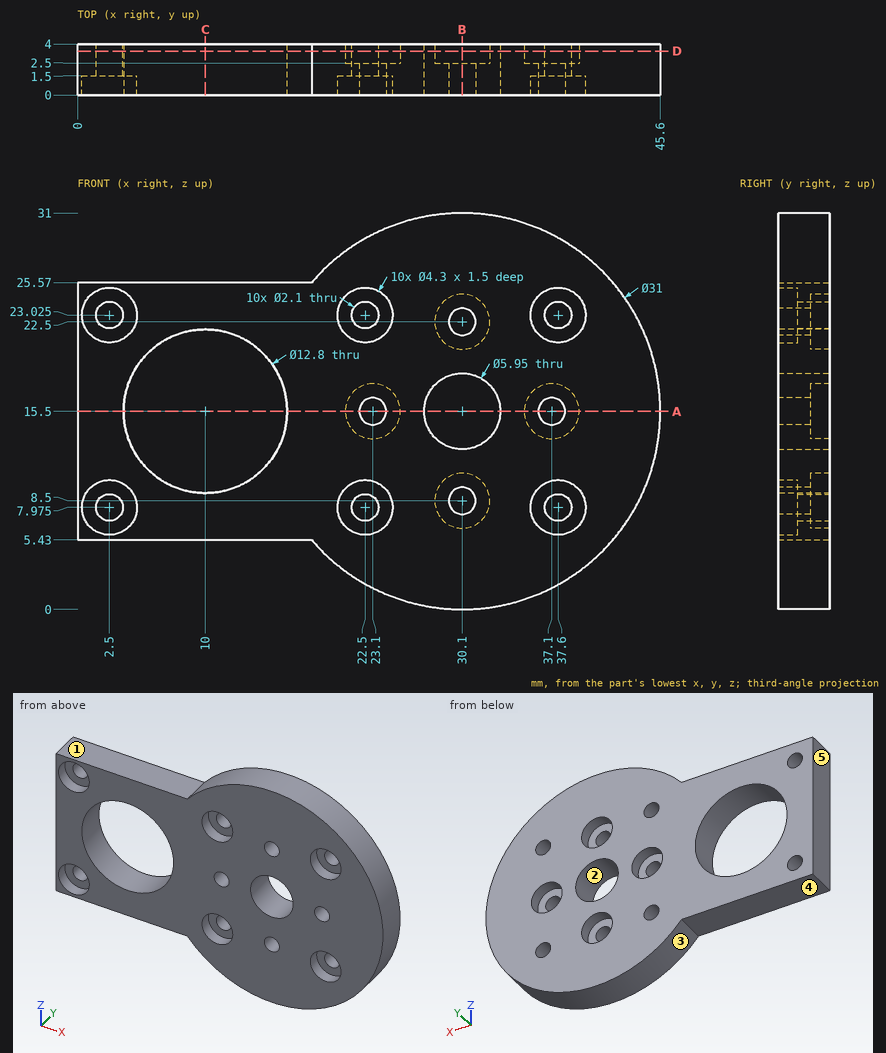
Geometry: see drawing. Coordinates: mm, zero at the bounding-box minimum. A direction names the side the tool comes from. Give positions to 0.01 mm unless a question says otherwise; leave off trailing zeros. Write each loop counter-clockwise with the first axis right and the second up, starting at its lowest first coordinate (ties: lowest second). Pieces come first, ordered by that corner, then holes. Notation, with made-up numbers: M 10,27 L 56,27 A34 cw 56,64 Z; hole C 81.5,51.25 d3. An arc over 180 degrees is marked long. Answer as a JSON object with one key per item and string values.
Q1. Contact query for flat-ended pins moving along their axis: P1, Ø1.3, axis at x = 37.5, z = 22, coming from the -Y side; P2, Ø1.3, axis at x = 2.5, z = 7.975, coming from the +Y side; P3, Ø2, axis at x = 29.5, z = 8, coming from the +Y side. Output: stop coordinate, or through.
Geometry check:
{"P1": "stops at y = 1.5", "P2": "passes through", "P3": "stops at y = 2.5"}
Q2. Cut plane B-B, the plane x = 30.1. Return the cut outline in (y, z) (3 decimals), then the cut area to 3 significant figures.
Geometry check:
{"outline": "M 0,0 L 4,0 L 4,6.35 L 2.5,6.35 L 2.5,7.45 L 0,7.45 Z; M 0,9.55 L 2.5,9.55 L 2.5,10.65 L 4,10.65 L 4,12.525 L 0,12.525 Z; M 0,18.475 L 4,18.475 L 4,20.35 L 2.5,20.35 L 2.5,21.45 L 0,21.45 Z; M 0,23.55 L 2.5,23.55 L 2.5,24.65 L 4,24.65 L 4,31 L 0,31 Z", "area": "76.8 mm^2"}
Q3. Ray query, line 1 along X through (y, z) = (0.8, 15.5) (3 decimals); line 2 along Z through (x, y) = (10, 3.25); line 3 along X through (y, z) = (0.2, 17.5). Return the intervals inside material, ascending.
Geometry check:
{"line 1": "x = 0 to 3.6, 16.4 to 22.05, 24.15 to 27.125, 33.075 to 36.05, 38.15 to 45.6", "line 2": "z = 5.43 to 9.1, 21.9 to 25.57", "line 3": "x = 0 to 3.92, 16.08 to 27.9, 32.3 to 45.47"}
Q4. Access query for the marked faces 4 and 5. Directions: +Z, -Z, +X, -X, +Y, -Y. A direction counts if a zero-diameter tool reaches every point of the face in a straight line with its end or side. Return the directions, or none.
Geometry check:
{"face 4": "-Z, -X, +Y, -Y", "face 5": "+Z, -Z, -X, +Y, -Y"}
Q5. Cut plane A-A, the plane z = 15.5. Return the cut outline in (x, y) (3 decimals).
Geometry check:
{"outline": "M 0,0 L 3.6,0 L 3.6,4 L 0,4 Z; M 16.4,0 L 22.05,0 L 22.05,2.5 L 20.95,2.5 L 20.95,4 L 16.4,4 Z; M 24.15,0 L 27.125,0 L 27.125,4 L 25.25,4 L 25.25,2.5 L 24.15,2.5 Z; M 33.075,0 L 36.05,0 L 36.05,2.5 L 34.95,2.5 L 34.95,4 L 33.075,4 Z; M 38.15,0 L 45.6,0 L 45.6,4 L 39.25,4 L 39.25,2.5 L 38.15,2.5 Z"}
Q6. Mould query, pull axis Z, two halves, no side actions, for the marked faces 1, 2 and 3. Classes: +Z half, -Z half, draft (parallel to the pull), parting line (faces both ways), or undercut.
Geometry check:
{"face 1": "+Z half", "face 2": "undercut", "face 3": "parting line"}
Q7. Cut plane C-C, the plane x = 10. Return the cut outline in (y, z), then the cut area to 3 significant figures.
Geometry check:
{"outline": "M 0,5.43 L 4,5.43 L 4,9.1 L 0,9.1 Z; M 0,21.9 L 4,21.9 L 4,25.57 L 0,25.57 Z", "area": "29.4 mm^2"}
Q8. Cut plane D-D, the plane y = 3.45. Count the separate pieces of the cut face and the enclosed holes in it, then the cut area to 3 significant figures.
Geometry check:
{"separate pieces": "1", "enclosed holes": "12", "area": "837 mm^2"}
